Check sheet for the modelled part. Datum: model origin and axes. Units: mm. Face numbers are marked on the shaded views. A direction names the side the tool comes from. Coordinates: 2 decimals unless noted, no trailing zeros. Loops run counter-clockwise (first coordinate to the right, second up) from the corner with the lowest first, then second, coordinate; pieces in that order, holes last. Notation, with made-up numbers: M 33.5,16 L 55.5,16 A28 ccw 55.5,39 Z; hole C 50.25,39.5 d9. An arc over 180 degrees is marked long. Use CSV: the item, a comma, the result in double quotes. Start each with the question number.
(1) Set-up check for the marked faces 1, 2 and 3: record each of +Z, -Z, +X, -X, +Y, -Y from which the full face is reachable in a straight line by a thin tool's end or side.
(2) Section check C-C on y = -1.5. Record the cut outline in (x, z).
(3) Section check A-A on y = 32. Give the number of separate pieces and of enclosed holes in the cut face, and give its area (3 significant figures).
(4) Scan lines: line 1 (Y direction, x = -27, z = -44); line 2 (Y direction, x = -6, z = 9); line 3 (Z direction, x = -3.5, y = 13.5). Record each from-to range of solid material in increasing order.
(5) Go/stop test with flat-tipped pins: pin 1 Ø6.5 at (x, z) = (-24.75, 24.75) entering from -Y; pin 2 Ø10 at (x, z) = (-26, -41) entering from -Y; pin 3 Ø8 at (x, z) = (-12.73, -12.73) entering from +Y; pin 4 Ø14.5 at (x, z) = (0, 0) entering from +Y. Record where each tip stops, or that it passes through.
from build123d import *

# Parameters (mm, degrees)
SKETCH1_R               = 60
BOSS_EXTRUDE1_DEPTH     = 46
SKETCH2_R               = 32
BOSS_EXTRUDE2_DEPTH     = 12
SKETCH3_R               = 31
BOSS_EXTRUDE3_DEPTH     = 3
SKETCH4_R               = 22.4
BOSS_EXTRUDE4_DEPTH     = 2
SKETCH6_R               = 12
CUT_EXTRUDE1_DEPTH      = 50
SKETCH8_R               = 2.5
CUT_EXTRUDE2_DEPTH      = 12
CUT_EXTRUDE3_DEPTH      = 103.78132126
CUT_EXTRUDE3_DEPTH_BACK = 103.78132126
SKETCH9_R               = 2.5
CHAMFER1_SIZE           = 2
CHAMFER2_SIZE           = 1


with BuildPart() as part:
    # Sketch1 → Boss-Extrude1 (new body)
    with BuildSketch(Plane(origin=(0, 0, 0), x_dir=(1, 0, 0), z_dir=(0, 1, 0))):
        with Locations(Location((0, 0, 0), (0, 0, 270))):
            Circle(SKETCH1_R)
    extrude(amount=BOSS_EXTRUDE1_DEPTH)

    # Sketch2 → Boss-Extrude2 (add)
    with BuildSketch(Plane.XZ):
        with Locations(Location((0, 0, 0), (0, 0, 270))):
            Circle(SKETCH2_R)
    extrude(amount=BOSS_EXTRUDE2_DEPTH)

    # Sketch3 → Boss-Extrude3 (add)
    with BuildSketch(Plane(origin=(0, 46, 0), x_dir=(1, 0, 0), z_dir=(0, 1, 0))):
        with Locations(Location((0, 0, 0), (0, 0, 270))):
            Circle(SKETCH3_R)
    extrude(amount=BOSS_EXTRUDE3_DEPTH)

    # Sketch4 → Boss-Extrude4 (add)
    with BuildSketch(Plane(origin=(0, 49, 0), x_dir=(1, 0, 0), z_dir=(0, 1, 0))):
        with Locations(Location((0, 0, 0), (0, 0, 270))):
            Circle(SKETCH4_R)
    extrude(amount=BOSS_EXTRUDE4_DEPTH)

    # Sketch6 → Cut-Extrude1 (cut)
    with BuildSketch(Plane(origin=(0, 51, 0), x_dir=(1, 0, 0), z_dir=(0, 1, 0))):
        with Locations(Location((0, 0, 0), (0, 0, 270))):
            Circle(SKETCH6_R)
    extrude(amount=-CUT_EXTRUDE1_DEPTH, mode=Mode.SUBTRACT)

    # Sketch8 → Cut-Extrude2 (cut)
    with BuildSketch(Plane(origin=(0, 51, 0), x_dir=(1, 0, 0), z_dir=(0, 1, 0))):
        with Locations(Location((0, 18, 0), (0, 0, 270))):
            Circle(SKETCH8_R)
        with Locations(Location((12.727922061, 12.727922061, 0), (0, 0, 270))):
            Circle(SKETCH8_R)
        with Locations(Location((18, 0, 0), (0, 0, 270))):
            Circle(SKETCH8_R)
        with Locations(Location((12.727922061, -12.727922061, 0), (0, 0, 270))):
            Circle(SKETCH8_R)
        with Locations(Location((0, -18, 0), (0, 0, 270))):
            Circle(SKETCH8_R)
        with Locations(Location((-12.727922061, -12.727922061, 0), (0, 0, 270))):
            Circle(SKETCH8_R)
        with Locations(Location((-18, 0, 0), (0, 0, 270))):
            Circle(SKETCH8_R)
        with Locations(Location((-12.727922061, 12.727922061, 0), (0, 0, 270))):
            Circle(SKETCH8_R)
    extrude(amount=-CUT_EXTRUDE2_DEPTH, mode=Mode.SUBTRACT)

    # Sketch9 → Cut-Extrude3 (cut, two sides: drawn at the far end of the back side and taken through both)
    with BuildSketch(Plane(origin=(0, 46, 0), x_dir=(1, 0, 0), z_dir=(0, 1, 0)).offset(-CUT_EXTRUDE3_DEPTH_BACK)):
        with Locations(Location((0, 35, 0), (0, 0, 270))):
            Circle(SKETCH9_R)
        with Locations(Location((24.748737342, 24.748737342, 0), (0, 0, 270))):
            Circle(SKETCH9_R)
        with Locations(Location((35, 0, 0), (0, 0, 270))):
            Circle(SKETCH9_R)
        with Locations(Location((24.748737342, -24.748737342, 0), (0, 0, 270))):
            Circle(SKETCH9_R)
        with Locations(Location((0, -35, 0), (0, 0, 270))):
            Circle(SKETCH9_R)
        with Locations(Location((-24.748737342, -24.748737342, 0), (0, 0, 270))):
            Circle(SKETCH9_R)
        with Locations(Location((-35, 0, 0), (0, 0, 270))):
            Circle(SKETCH9_R)
        with Locations(Location((-24.748737342, 24.748737342, 0), (0, 0, 270))):
            Circle(SKETCH9_R)
    extrude(amount=CUT_EXTRUDE3_DEPTH + CUT_EXTRUDE3_DEPTH_BACK, mode=Mode.SUBTRACT)

    # Chamfer1
    chamfer1_edges = [part.edges().sort_by_distance(p)[0] for p in [
        (0, 0, -60),
        (0, 46, -60),
    ]]
    chamfer(chamfer1_edges, length=CHAMFER1_SIZE)

    # Chamfer2
    chamfer2_edges = [part.edges().sort_by_distance(p)[0] for p in [
        (0, 49, -31),
        (0, -12, 32),
    ]]
    chamfer(chamfer2_edges, length=CHAMFER2_SIZE)


solid = part.part
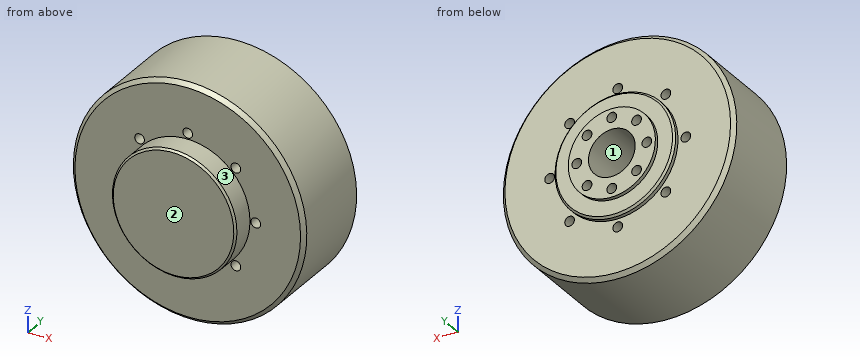
Outcome:
1,face 1,"+Y"
1,face 2,"+Z, -Z, +X, -X, -Y"
1,face 3,"-Y"
2,outline,"C 0,0 d64"
3,separate pieces,"1"
3,enclosed holes,"9"
3,area,"10,700 mm²"
4,line 1,"y = 0 to 46"
4,line 2,"y = -12 to 1"
4,line 3,"z = -59.9 to -11.48, 11.48 to 59.9"
5,pin 1,"stops at y = -11.25"
5,pin 2,"stops at y = 0"
5,pin 3,"stops at y = 51"
5,pin 4,"stops at y = 1"
